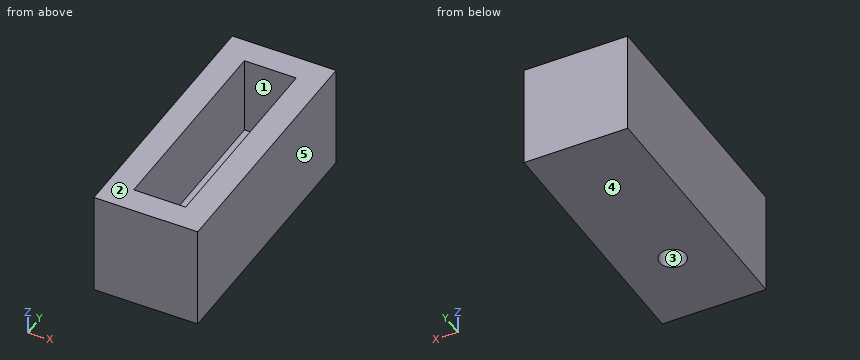
from build123d import *

# Parameters (mm, degrees)
F0_W     = 10
F0_H     = 10
F1_DEPTH = 12.5
F2_T     = -2.5
F3_R     = 1.25
F4_DEPTH = 10.001


with BuildPart() as f1:
    # F0 (on Front) → F1 (new body, symmetric)
    with BuildSketch(Plane.XZ):
        Rectangle(F0_W, F0_H)
    extrude(amount=F1_DEPTH, both=True)

    # F2
    f2_openings = [f1.faces().sort_by_distance(p)[0] for p in [
        (0, 0, 5),
    ]]
    offset(amount=F2_T, openings=f2_openings)

    # F3 (on face) → F4 (cut, through all)
    with BuildSketch(Plane(origin=(0, 0, -5), x_dir=(1, 0, 0), z_dir=(0, 0, -1))):
        with Locations((0, 5)):
            Circle(F3_R)
    extrude(amount=-F4_DEPTH, mode=Mode.SUBTRACT)


solid = f1.part
Here's how the part is built. I have some questions about the finished solid (model axes, mm). Face numbers are marked on the shaded views. A direction names the side the tool comes from. Round coordinates to 2 decimals unless told otherwise and drop trailing zeros. Loops run counter-clockwise (first coordinate to the right, second up) from the corner with the lowest first, then second, coordinate; pieces in that order, holes last.
1. If I drill on line 1 along Y through (x, z) = (0, -3.85); line 2 along Y through (x, z) = (-0.5, 3); line 3 along X through (y, z) = (0.25, -1.75), over which ranges is the centre line in solid material (lowest first)?
Answer list:
line 1: y = -12.5 to -6.25, -3.75 to 12.5
line 2: y = -12.5 to -10, 10 to 12.5
line 3: x = -5 to -2.5, 2.5 to 5
2. If we section it at A-A on x = 0: Write out the boundary of the cut face in (y, z).
Answer list:
outline: (-12.5, -5) - (-6.25, -5) - (-6.25, -2.5) - (-10, -2.5) - (-10, 5) - (-12.5, 5) - close; (-3.75, -5) - (12.5, -5) - (12.5, 5) - (10, 5) - (10, -2.5) - (-3.75, -2.5) - close
3. If we section it at C-C on y = -5: Write out the boundary of the cut face in (x, z).
Answer list:
outline: (-5, -5) - (-1.25, -5) - (-1.25, -2.5) - (-2.5, -2.5) - (-2.5, 5) - (-5, 5) - close; (1.25, -5) - (5, -5) - (5, 5) - (2.5, 5) - (2.5, -2.5) - (1.25, -2.5) - close
4. Which directions (+Z, -Z, +X, -X, +Y, -Y) give clear straight access to the entire face, cutting with the end or side of a thin tool? Please do the marked faces 1 and 2.
Answer list:
face 1: +Z
face 2: +Z, +X, -X, +Y, -Y
5. We'd pull the mould along X, two halves only. Please class the marked faces 3, 4 and 5: +X half, -X half, draft (parallel to the pull), parting line (faces both ways), or undercut.
Answer list:
face 3: undercut
face 4: draft
face 5: +X half
6. If we section it at D-D on x = -1.5: Write out the boundary of the cut face in (y, z), plus the area to 3 significant figures.
Answer list:
outline: (-12.5, -5) - (12.5, -5) - (12.5, 5) - (10, 5) - (10, -2.5) - (-10, -2.5) - (-10, 5) - (-12.5, 5) - close
area: 100 mm2
7. If we section it at B-B on z = 4.75: Write out the boundary of the cut face in (x, y), plus the area to 3 significant figures.
Answer list:
outline: (-5, -12.5) - (5, -12.5) - (5, 12.5) - (-5, 12.5) - close; hole (-2.5, -10) - (2.5, -10) - (2.5, 10) - (-2.5, 10) - close
area: 150 mm2
